from build123d import *

# Parameters (mm, degrees)
BOSS_EXTRUDE1_DEPTH = 1
SKETCH2_R           = 2.5
BOSS_EXTRUDE2_DEPTH = 1


with BuildPart() as part:
    # Sketch1 → Boss-Extrude1 (new body)
    with BuildSketch(Plane(origin=(0, 0, 0), x_dir=(1, 0, 0), z_dir=(0, 1, 0))):
        Polygon((9.725, 200), (4.275, 200), (0, 200), (4.275, 0), (9.725, 0), (14, 200), align=None)
    extrude(amount=BOSS_EXTRUDE1_DEPTH)

    # Sketch2 → Boss-Extrude2 (add)
    with BuildSketch(Plane.XZ):
        with BuildLine():
            Line((0, -200), (14, -200))
            Line((14, -200), (14, -213))
            ThreePointArc((14, -213), (7, -220), (0, -213))
            Line((0, -213), (0, -200))
        make_face()
        with Locations(Location((7, -213, 0), (0, 0, 270))):
            Circle(SKETCH2_R, mode=Mode.SUBTRACT)
    extrude(amount=-BOSS_EXTRUDE2_DEPTH)


solid = part.part
Could you check a few things on this model? Use its own coordinates, in mm. Give positions to 0.01 mm unless a question says otherwise; leave off trailing zeros. Order: outer loops, then holes, each group sorted by start corner. A loop starts at its lowest first (then second) coordinate and runs counter-clockwise, first axis right, second up.
1. Thinking about a two-plate mould opening in Z: for faces 1 (the cylindrical face through (7.15, 0.49, -220)), 2 (the cylindrical face through (6.04, 0.49, -215.31)), 3 (the flat face through (7, 0, -133)), which applies, +Z half, -Z half, draft (parallel to the pull), parting line (faces both ways), or undercut?
Answers below:
face 1: -Z half
face 2: undercut
face 3: draft
2. Suppose I cut it at D-D (z = -117). Write out the boundary of the cut face in (x, y), plus the area to 3 significant figures.
Answers below:
outline: (1.77, 0) - (12.23, 0) - (12.23, 1) - (1.77, 1) - close
area: 10.5 mm2
3. Suppose I cut it at C-C (z = -49.5). Write out the boundary of the cut face in (x, y), plus the area to 3 significant figures.
Answers below:
outline: (3.22, 0) - (10.78, 0) - (10.78, 1) - (3.22, 1) - close
area: 7.57 mm2
4. I need wall thicknesses on L1, parallel to X at y = 0.25, z = -213; L2, parallel to Z at x = 9, y = 0.25; L3, parallel to Z at x = 5.75, y = 0.35. Which ranges of each line are inside material? Lowest first, please.
Answers below:
L1: x = 0 to 4.5, 9.5 to 14
L2: z = -219.71 to -214.5, -211.5 to 0
L3: z = -219.89 to -215.17, -210.83 to 0
5. Suppose I cut it at B-B (y = 0.3). Write out the boundary of the cut face in (x, z) (3 decimals).
Answers below:
outline: (0, -213) arc R7 ccw to (14, -213) - (14, -200) - (9.725, 0) - (4.275, 0) - (0, -200) - close; hole circle Ø5 at (7, -213)
6. Suppose I cut it at A-A (x = 7). Write out the boundary of the cut face in (y, z), plus the area to 3 significant figures.
Answers below:
outline: (0, -220) - (1, -220) - (1, -215.5) - (0, -215.5) - close; (0, -210.5) - (1, -210.5) - (1, 0) - (0, 0) - close
area: 215 mm2
